```python
from build123d import *

# Parameters (mm, degrees)
SKETCH1_R           = 1.5
BOSS_EXTRUDE1_DEPTH = 4
FILLET1_R           = 2


with BuildPart() as part:
    # Sketch1 → Boss-Extrude1 (new body)
    with BuildSketch(Plane.XY):
        with BuildLine():
            Line((20.430139316, 13), (119.569860684, 13))
            ThreePointArc((119.569860684, 13), (132.344758657, 10.310849901), (142.951440202, 2.699814945))
            ThreePointArc((142.951440202, 2.699814945), (142.64957914, -2.996619826), (136.959055493, -2.598587405))
            ThreePointArc((136.959055493, -2.598587405), (129.548246583, 3.008962434), (120.470775938, 5))
            Line((120.470775938, 5), (19.529224062, 5))
            ThreePointArc((19.529224062, 5), (10.451753417, 3.008962434), (3.040944507, -2.598587405))
            ThreePointArc((3.040944507, -2.598587405), (-2.64957914, -2.996619826), (-2.951440202, 2.699814945))
            ThreePointArc((-2.951440202, 2.699814945), (7.655241343, 10.310849901), (20.430139316, 13))
        make_face()
        Circle(SKETCH1_R, mode=Mode.SUBTRACT)
        with Locations(Location((140, 0, 0), (0, 0, 180))):
            Circle(SKETCH1_R, mode=Mode.SUBTRACT)
    extrude(amount=BOSS_EXTRUDE1_DEPTH)

    # Fillet1
    fillet1_edges = [part.edges().sort_by_distance(p)[0] for p in [
        (10.451753417, 3.008962434, 4),
        (-2.64957914, -2.996619826, 4),
        (7.655241343, 10.310849901, 4),
        (70, 13, 4),
        (132.344758657, 10.310849901, 4),
        (142.64957914, -2.996619826, 4),
        (129.548246583, 3.008962434, 4),
        (10.451753417, 3.008962434, 0),
        (-2.64957914, -2.996619826, 0),
        (7.655241343, 10.310849901, 0),
        (70, 13, 0),
        (132.344758657, 10.310849901, 0),
        (142.64957914, -2.996619826, 0),
        (129.548246583, 3.008962434, 0),
        (70, 5, 4),
        (70, 5, 0),
    ]]
    fillet(fillet1_edges, radius=FILLET1_R - 0.0001)  # a hair under: the kernel refuses the full size


solid = part.part
```
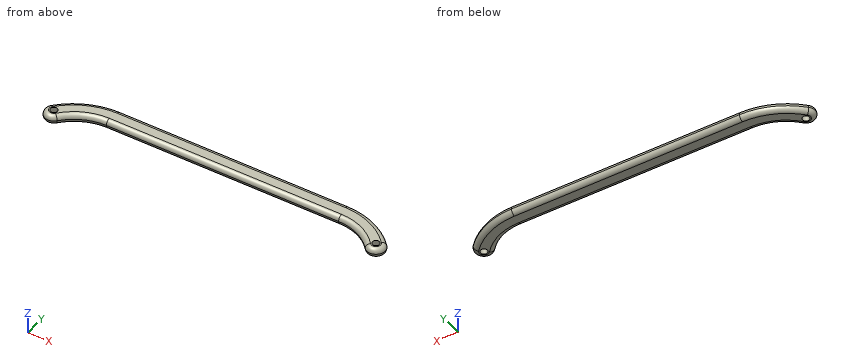
Work out the finished part from the listing and answer in its coordinate system (mm). Give positions to 0.01 mm unless a question says otherwise; leave off trailing zeros. Loops run counter-clockwise (first coordinate to the right, second up) from the corner with the lowest first, then second, coordinate; pieces in that order, holes last. Notation, with made-up numbers: (43, 19.5) -> (78, 19.5) arc R16 cw to (78, 46.5) -> close; hole circle Ø4 at (47.25, 37). An arc over 180 degrees is marked (long way). Write item = value, one per line. Start each with the question number.
(1) Find section C-C on y = 0. Give the number of separate pieces and of enclosed holes in the cut face, and give its area (3 significant figures).
(2) Find section B-B on z = 3.35. Give the vertices of the cut face in (x, y).
(3) Find the intervals of material crossed by probe 1 along X at (y, z) = (0.5, 2.65); probe 2 along X at (y, z) = (0.5, 2.1); probe 3 along X at (y, z) = (2, 1.05), in increasing order. Write a range as from..to.
From the geometry:
q1.separate_pieces = 4
q1.enclosed_holes = 0
q1.area = 44.8 mm^2
q2.outline = (-2.56, 2.35) arc R3.48 ccw (long way) to (2.64, -2.26) arc R22.21 cw to (19.53, 5.52) -> (120.47, 5.52) arc R22.21 cw to (137.36, -2.26) arc R3.48 ccw (long way) to (142.56, 2.35) arc R31.16 ccw to (119.57, 12.48) -> (20.43, 12.48) arc R31.16 ccw to start; hole circle Ø3 at (0, 0); hole circle Ø3 at (140, 0)
q3.probe_1 = -3.86..-1.41, 1.41..6.13, 133.87..138.59, 141.41..143.86
q3.probe_2 = -3.97..-1.41, 1.41..6.3, 133.7..138.59, 141.41..143.97
q3.probe_3 = -3.18..8.06, 131.94..143.18
